CAD build for the part. Positions are in the model's coordinates, mm. Face numbers are marked on the shaded views. A direction names the side the tool comes from. Round coordinates to 2 decimals unless told otherwise and drop trailing zeros. Loops run counter-clockwise (first coordinate to the right, second up) from the corner with the lowest first, then second, coordinate; pieces in that order, holes last. Notation, with made-up numbers: M -20.75,-20.75 L 38.25,-20.75 A26 cw 38.25,0.25 Z; hole C 21,83 d5. An arc over 180 degrees is marked long. Use a Markdown table: item, result. Add a question column.
(1) Which spindle directions (+Z, -Z, +X, -X, +Y, -Y) get a long thin tool onto all of the face, cutting with end or side? Do the marked faces 4 and 5. Say none if no direction does.
(2) Band-saw the part on A-A, the plane z = 42.5. Write the cut outline in (x, y).
(3) Two-plate mould, pull along Z, no slides. Class the marked faces 1, 2 and 3: released by +Z, released by -Z, zero draft, split by the parting line, or undercut.
(4) Band-saw the part on B-B, the plane x = 12. Write the cut outline in (y, z).
(5) Wall check: L1, parallel to X at y = 131, z = 10; L2, parallel to Z at x = 5, y = 120; L3, parallel to Z at x = 5, y = 139. Give the ranges that are in metal, low to high.
(6) Flat gauge pins, fed straight in: P1, Ø2, axis at x = 29, y = 66, coming from the +Z side; P2, Ø12, axis at x = 32, y = 98, coming from the -Z side; P3, Ø5, axis at x = 18.5, y = 133, coming from the -Z side. Where does each tip first touch, or does it go through?
from build123d import *

# Parameters (mm, degrees)
BOSS_EXTRUDE1_DEPTH = 40
SKETCH2_R           = 3
CUT_EXTRUDE1_DEPTH  = 40
CUT_EXTRUDE2_DEPTH  = 40
FILLET1_R           = 5


with BuildPart() as part:
    # Sketch1 → Boss-Extrude1 (new body)
    with BuildSketch(Plane(origin=(0, 0, 0), x_dir=(0, 0, -1), z_dir=(1, 0, 0))):
        Polygon((-20, 150), (20, 150), (35, 5), (50, 5), (50, 0), (15, 0), (0, 70.528805369), (-15, 0), (-50, 0), (-50, 5), (-35, 5), align=None)
    extrude(amount=BOSS_EXTRUDE1_DEPTH)

    # Sketch2 → Cut-Extrude1 (cut)
    with BuildSketch(Plane(origin=(0, 5, 0), x_dir=(1, 0, 0), z_dir=(0, 1, 0))):
        with Locations(Location((20, 42.5, 0), (0, 0, 270))):
            Circle(SKETCH2_R)
        with Locations(Location((20, -42.5, 0), (0, 0, 270))):
            Circle(SKETCH2_R)
    extrude(amount=-CUT_EXTRUDE1_DEPTH, mode=Mode.SUBTRACT)

    # Sketch3 → Cut-Extrude2 (cut)
    with BuildSketch(Plane(origin=(0, 150, 0), x_dir=(1, 0, 0), z_dir=(0, 1, 0))):
        with BuildLine():
            ThreePointArc((35, -8), (33.585786438, -8.585786438), (33, -10))
            Line((33, -10), (35, -10))
            Line((35, -10), (35, -8))
        make_face()
        with BuildLine():
            Line((35, -10), (33, -10))
            ThreePointArc((33, -10), (35, -12), (37, -10))
            ThreePointArc((37, -10), (36.414213562, -8.585786438), (35, -8))
            Line((35, -8), (35, -10))
        make_face()
        with BuildLine():
            ThreePointArc((33, 10), (33.585786438, 8.585786438), (35, 8))
            Line((35, 8), (35, 10))
            Line((35, 10), (33, 10))
        make_face()
        with BuildLine():
            Line((35, 10), (35, 8))
            ThreePointArc((35, 8), (36.414213562, 8.585786438), (37, 10))
            ThreePointArc((37, 10), (35, 12), (33, 10))
            Line((33, 10), (35, 10))
        make_face()
        with BuildLine():
            ThreePointArc((7, 10), (3.585786438, 11.414213562), (5, 8))
            Line((5, 8), (5, 10))
            Line((5, 10), (7, 10))
        make_face()
        with BuildLine():
            Line((5, 10), (5, 8))
            ThreePointArc((5, 8), (6.414213562, 8.585786438), (7, 10))
            Line((7, 10), (5, 10))
        make_face()
        with BuildLine():
            Line((5, -8), (5, -10))
            Line((5, -10), (7, -10))
            ThreePointArc((7, -10), (6.414213562, -8.585786438), (5, -8))
        make_face()
        with BuildLine():
            Line((7, -10), (5, -10))
            Line((5, -10), (5, -8))
            ThreePointArc((5, -8), (3.585786438, -11.414213562), (7, -10))
        make_face()
    extrude(amount=-CUT_EXTRUDE2_DEPTH, mode=Mode.SUBTRACT)

    # Fillet1
    fillet1_edges = [part.edges().sort_by_distance(p)[0] for p in [
        (0, 2.5, -50),
        (0, 35.264402685, -7.5),
        (0, 35.264402685, 7.5),
        (40, 77.5, 27.5),
        (0, 2.5, 50),
        (0, 77.5, 27.5),
        (0, 77.5, -27.5),
        (40, 2.5, 50),
        (40, 35.264402685, 7.5),
        (40, 35.264402685, -7.5),
        (40, 2.5, -50),
        (40, 77.5, -27.5),
    ]]
    fillet(fillet1_edges, radius=FILLET1_R)


solid = part.part
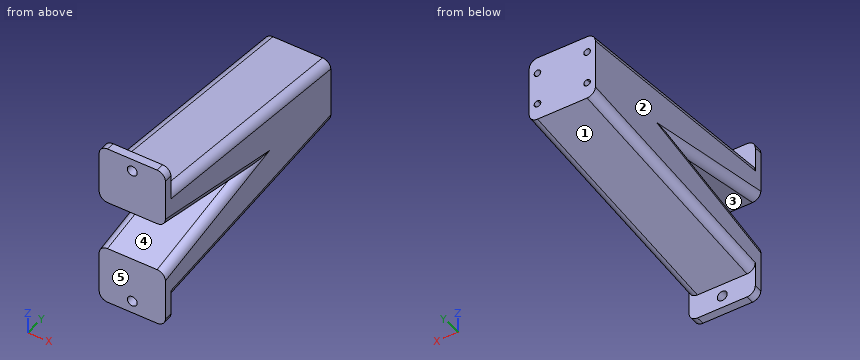
Return value:
| question | item | result |
|---|---|---|
| 1 | face 4 | +X, -X, -Y |
| 1 | face 5 | +Z, -Z, +X, -X, -Y |
| 2 | outline | M 0,0 L 17,0 L 17,5 L 0,5 Z; M 23,0 L 40,0 L 40,5 L 23,5 Z |
| 3 | face 1 | released by -Z |
| 3 | face 2 | zero draft |
| 3 | face 3 | undercut |
| 4 | outline | M 0,-50 L 5,-50 L 5,-35 L 150,-20 L 150,20 L 5,35 L 5,50 L 0,50 L 0,15 L 70.53,0 L 0,-15 Z |
| 5 | L1 | 0 to 3, 7 to 33, 37 to 40 |
| 5 | L2 | -23.1 to -12, -8 to 8, 12 to 23.1 |
| 5 | L3 | -21.14 to -12, -8 to 8, 12 to 21.14 |
| 6 | P1 | z = 28.79 |
| 6 | P2 | z = -26 |
| 6 | P3 | z = -22.02 |
